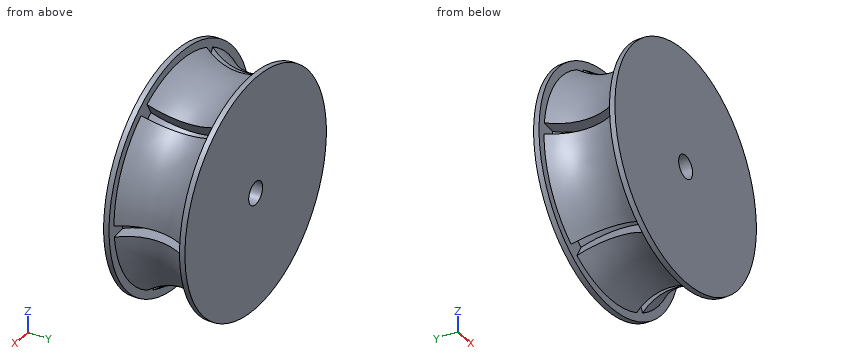
```python
from build123d import *

# Parameters (mm, degrees)
SKETCH3_R          = 6.35
CUT_EXTRUDE1_DEPTH = 102.849420847
CUT_REVOLVE5_ANGLE = 6
CIRPATTERN1_COUNT  = 6


with BuildPart() as part:
    # Sketch1 → Revolve1 (revolve)
    with BuildSketch(Plane(origin=(0, 0, 0), x_dir=(0, 0, -1), z_dir=(1, 0, 0))):
        with BuildLine():
            Line((-60.072805913, 19.55), (-64.572805913, 19.55))
            Line((-64.572805913, 19.55), (-64.572805913, 22.55))
            Line((-64.572805913, 22.55), (0, 22.55))
            Line((0, 22.55), (0, -22.55))
            Line((0, -22.55), (-64.572805913, -22.55))
            Line((-64.572805913, -22.55), (-64.572805913, -19.55))
            Line((-64.572805913, -19.55), (-60.072805913, -19.55))
            ThreePointArc((-60.072805913, -19.55), (-53.34, 0), (-60.072805913, 19.55))
        make_face()
    revolve(axis=Axis((0, 22.55, 0), (0, -1, 0)))

    # Sketch3 → Cut-Extrude1 (cut, through all)
    with BuildSketch(Plane(origin=(0, 22.55, 0), x_dir=(1, 0, 0), z_dir=(0, 1, 0))):
        with Locations(Location((0, 0, 0), (0, 0, 270))):
            Circle(SKETCH3_R)
    extrude(amount=-CUT_EXTRUDE1_DEPTH, mode=Mode.SUBTRACT)

    # Sketch4 → Cut-Revolve5 (revolve, cut)
    with BuildSketch(Plane.XY):
        with BuildLine():
            Line((-60.072805913, 19.55), (-52.452805913, 19.55))
            ThreePointArc((-52.452805913, 19.55), (-45.72, 0), (-52.452805913, -19.55))
            Line((-52.452805913, -19.55), (-60.072805913, -19.55))
            ThreePointArc((-60.072805913, -19.55), (-53.34, 0), (-60.072805913, 19.55))
        make_face()
    cut_revolve5 = revolve(axis=Axis((0, 0, 0), (0, 1, 0)), revolution_arc=CUT_REVOLVE5_ANGLE, mode=Mode.SUBTRACT)

    # CirPattern1: Cut-Revolve5 ×6 about axis
    cirpattern1_axis = Axis((0, 0, 0), (0, 1, 0))
    for i in range(1, CIRPATTERN1_COUNT):
        add(cut_revolve5.rotate(cirpattern1_axis, i * 360 / CIRPATTERN1_COUNT), mode=Mode.SUBTRACT)


solid = part.part
```
Geometry: final body of the model. Coordinates: model frame, mm. Round coordinates to 2 decimals unless told otherwise and drop trailing zeros. Write each loop counter-clockwise with the first axis right and the second up, starting at its lowest first coordinate (ties: lowest second). Pieces come first, ordered by that corner, then holes.
Item 1: Pin query (flat end, axial travel): P1, Ø2, axis at y = -4, z = -40.5, coming from the -X side; P2, Ø10, axis at x = 40, y = 2, coming from the +Z side; P3, Ø1.5, axis at y = 3.5, z = -13, coming from the +X side; P4, Ø16.5, axis at x = 0, z = 0, coming from the +Y side. Return the tip coordinate at first contact, or that it passes through.
Item 2: Material intervals for L1, parallel to X at y = -9.5, z = -42.5; L2, parallel to Z at x = -19, y = 6; L3, parallel to Z at x = 25, y = 14, sorted ascending.
Item 3: Section query A-A (x = 0). Return loops of the section in (y, z), plus the area to 3 significant figures.
Item 4: Section query C-C (y = 10). Return loops of the section in (x, z).
Item 5: Section query B-B (y = -14). Return loops of the section in (x, z) (3 decimals), plus the area to 3 significant figures.
Completed:
1. P1: stops at x = -36.24
1. P2: stops at z = 40.36
1. P3: stops at x = 52.13
1. P4: stops at y = 22.55
2. L1: x = -34.59 to -30.88, -24.54 to 20.47, 24.54 to 34.59
2. L2: z = -50.45 to 42.21, 42.67 to 50.45
2. L3: z = -43.3 to 42.11, 43.3 to 50.77
3. outline: (-22.55, -64.57) - (-19.55, -64.57) - (-19.55, -60.07) arc R31.75 cw to (19.55, -60.07) - (19.55, -64.57) - (22.55, -64.57) - (22.55, -6.35) - (-22.55, -6.35) - close; (-22.55, 6.35) - (22.55, 6.35) - (22.55, 64.57) - (19.55, 64.57) - (19.55, 60.07) arc R31.75 cw to (-19.55, 60.07) - (-19.55, 64.57) - (-22.55, 64.57) - close
3. area: 4,540 mm2
4. outline: (-54.96, 0) arc R54.96 ccw to (-32.3, -44.46) - (-27.82, -38.3) arc R47.34 ccw to (-23.67, -40.99) - (-27.48, -47.59) arc R54.96 ccw to (22.35, -50.2) - (19.25, -43.24) arc R47.34 ccw to (23.67, -40.99) - (27.48, -47.59) arc R54.96 ccw to (54.65, -5.74) - (47.08, -4.95) arc R47.34 ccw to (47.34, 0) - (54.96, 0) arc R54.96 ccw to (32.3, 44.46) - (27.82, 38.3) arc R47.34 ccw to (23.67, 40.99) - (27.48, 47.59) arc R54.96 ccw to (-22.35, 50.2) - (-19.25, 43.24) arc R47.34 ccw to (-23.67, 40.99) - (-27.48, 47.59) arc R54.96 ccw to (-54.65, 5.74) - (-47.08, 4.95) arc R47.34 ccw to (-47.34, 0) - close; hole circle Ø12.7 at (0, 0)
5. outline: (-56.593, 0) arc R56.593 ccw to (-33.265, -45.785) - (-28.786, -39.62) arc R48.973 ccw to (-24.487, -42.412) - (-28.297, -49.011) arc R56.593 ccw to (23.019, -51.701) - (19.919, -44.739) arc R48.973 ccw to (24.487, -42.412) - (28.297, -49.011) arc R56.593 ccw to (56.283, -5.916) - (48.705, -5.119) arc R48.973 ccw to (48.973, 0) - (56.593, 0) arc R56.593 ccw to (33.265, 45.785) - (28.786, 39.62) arc R48.973 ccw to (24.487, 42.412) - (28.297, 49.011) arc R56.593 ccw to (-23.019, 51.701) - (-19.919, 44.739) arc R48.973 ccw to (-24.487, 42.412) - (-28.297, 49.011) arc R56.593 ccw to (-56.283, 5.916) - (-48.705, 5.119) arc R48.973 ccw to (-48.973, 0) - close; hole circle Ø12.7 at (0, 0)
5. area: 9,680 mm2
